The figure shows three views and two pictorial views of one solid part (mm, origin at its lowest corner). Answer the questions. Give positions to 0.01 mm unless a question says otherwise; leave off trailing zeros. Loops run counter-clockwise (first coordinate to the right, second up) from the corner with the lowest first, then second, coordinate; pieces in that order, holes last. Notation, with made-up numbers: (54.5, 75.5) - (64.5, 75.5) arc R24 cw to (64.5, 86.5) - close; hole circle Ø3 at (65.5, 21.25). An arc over 180 degrees is marked (long way). One line per question, with ' | ' between items.
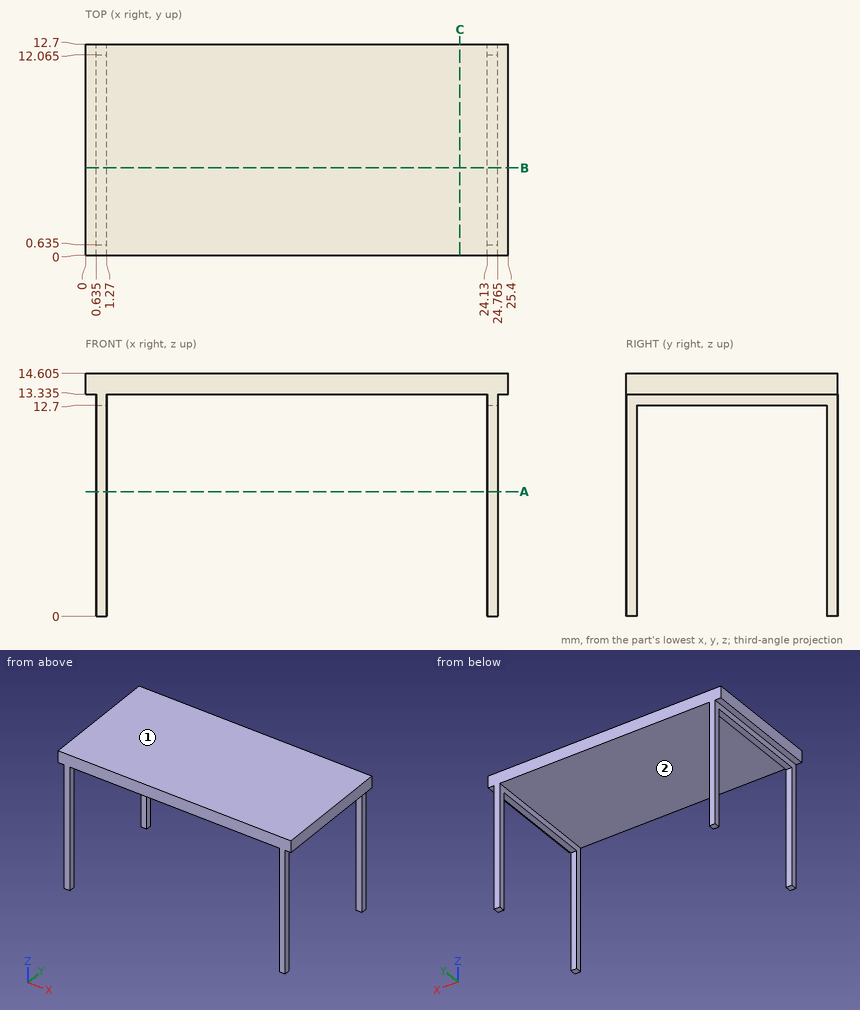
1. Determine the mould class of the marked faces 1 and 2 for opening direction X: +X half, -X half, draft (parallel to the pull), parting line (faces both ways), or undercut.
Evaluation:
face 1: draft | face 2: undercut
2. Find section C-C on x = 22.5. Write down the section's boundary in (y, z) (3 decimals).
Evaluation:
outline: (0, 13.335) - (12.7, 13.335) - (12.7, 14.605) - (0, 14.605) - close
3. Find section B-B on y = 5.25. Write down the section's boundary in (x, z) (3 decimals).
Evaluation:
outline: (0, 13.335) - (0.635, 13.335) - (0.635, 12.7) - (1.27, 12.7) - (1.27, 13.335) - (24.13, 13.335) - (24.13, 12.7) - (24.765, 12.7) - (24.765, 13.335) - (25.4, 13.335) - (25.4, 14.605) - (0, 14.605) - close
4. Flat-ended cylindrical pins translate along their axes: pin 1 (4 mm diameter, centred on x = 22, y = 3, fed in from -Z) (3 decimals); pin 2 (1 mm diameter, centred on x = 22.5, z = 9.5, fed in from -Y); pin 3 (1 mm diameter, centred on y = 4, z = 12.5, fed in from +X) (3 decimals); pin 4 (0.5 mm diameter, centred on x = 1, y = 5.5, fed in from -Z). Find the tip coordinate at first contact, or state that the pin passes through.
Evaluation:
pin 1: z = 13.335 | pin 2: through | pin 3: x = 24.765 | pin 4: z = 12.7
5. Consider L1, parallel to Z at x = 3.75, y = 6.5 (3 decimals). Determine where the line is inside the solid, lowest interval first.
Evaluation:
L1: 13.335 to 14.605
6. Find section A-A on z = 7.5. Write down the section's boundary in (x, y) (3 decimals), then the cut area to 3 significant figures.
Evaluation:
outline: (0.635, 0) - (1.27, 0) - (1.27, 0.635) - (0.635, 0.635) - close; (0.635, 12.065) - (1.27, 12.065) - (1.27, 12.7) - (0.635, 12.7) - close; (24.13, 0) - (24.765, 0) - (24.765, 0.635) - (24.13, 0.635) - close; (24.13, 12.065) - (24.765, 12.065) - (24.765, 12.7) - (24.13, 12.7) - close | area: 1.61 mm2
